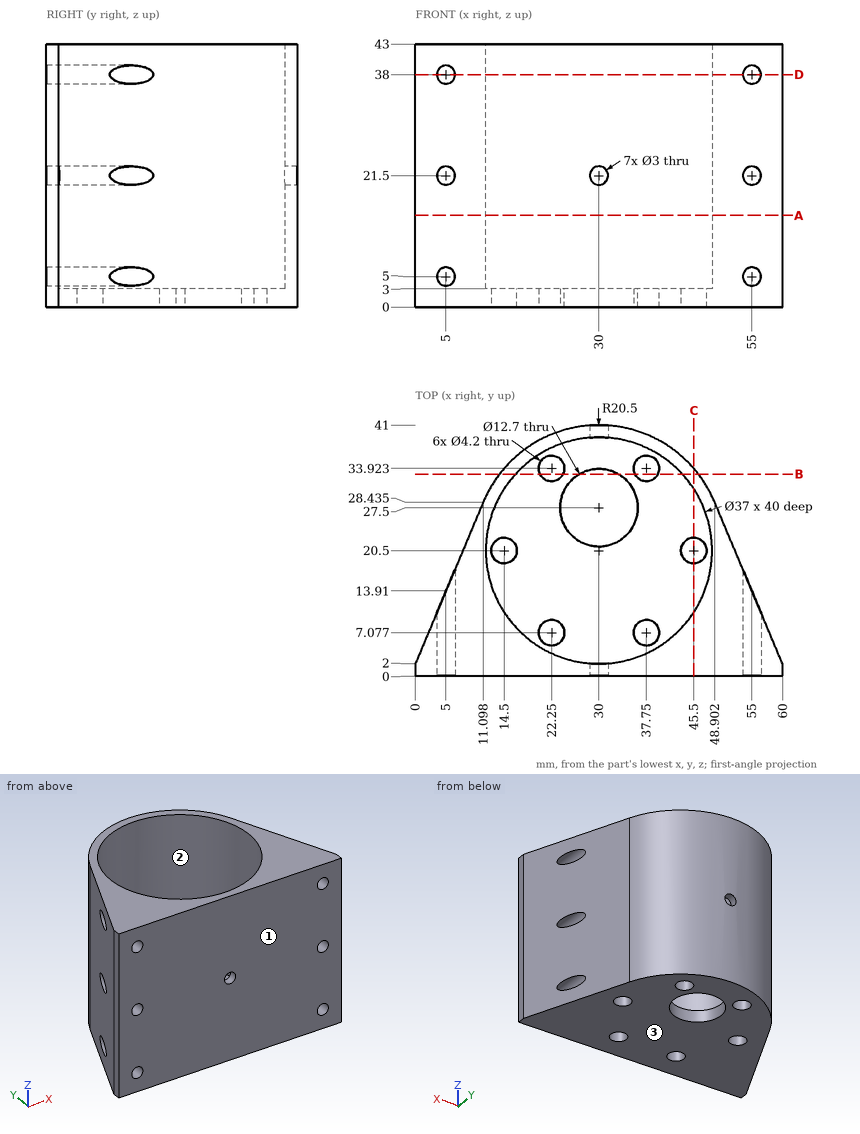
Design review of the part shown in the three views and the two pictorial views. Dimensions are in mm from the part's minimum x, y and z. Round coordinates to 2 decimals unless told otherwise and drop trailing zeros. Loops run counter-clockwise (first coordinate to the right, second up) from the corner with the lowest first, then second, coordinate; pieces in that order, holes last. Notation, with made-up numbers: M 48.5,-21 L 66.5,-21 A34 cw 66.5,16 Z; hole C 7,88 d6. An arc over 180 degrees is marked long. Put each result on its own line as item: value.
Q1. Consider section C-C, the plane x = 45.5. Give the boundary of the cut face in (y, z), then the cut area to 3 significant figures.
Result set:
outline: M 0,0 L 18.4,0 L 18.4,3 L 10.4,3 L 10.4,43 L 0,43 Z; M 22.6,0 L 33.92,0 L 33.92,43 L 30.6,43 L 30.6,3 L 22.6,3 Z
area: 638 mm²
Q2. Consider section B-B, the plane y = 33. Give the boundary of the cut face in (x, z).
Result set:
outline: M 13.75,0 L 20.36,0 L 20.36,3 L 16.36,3 L 16.36,43 L 13.75,43 Z; M 24.14,0 L 26.83,0 L 26.83,3 L 24.14,3 Z; M 33.17,0 L 35.86,0 L 35.86,3 L 33.17,3 Z; M 39.64,0 L 46.25,0 L 46.25,43 L 43.64,43 L 43.64,3 L 39.64,3 Z
Q3. To check wall thickness, follow L1, parallel to Z at x = 55, y = 11; L2, parallel to X at y = 5, z = 37 (1 decimal); L3, parallel to X at y = 7.25, z = 21.5 (1 decimal). State the ranges of each line that lie inside material, in increasing order.
Result set:
L1: z = 0 to 3.5, 6.5 to 20, 23 to 36.5, 39.5 to 43
L2: x = 1.3 to 3.9, 6.1 to 19.9, 40.1 to 53.9, 56.1 to 58.7
L3: x = 2.2 to 3.5, 6.5 to 17.1, 42.9 to 53.5, 56.5 to 57.8
Q4. Consider section A-A, the plane z = 15. Give the boundary of the cut face in (x, y) (1 decimal).
Result set:
outline: M 0,0 L 60,0 L 60,2 L 48.9,28.4 A20.5 ccw 11.1,28.4 L 0,2 Z; hole C 30,20.5 d37
Q5. Consider section D-D, the plane z = 38. Give the boundary of the cut face in (x, y) (1 decimal), then the cut area to 3 significant figures.
Result set:
outline: M 0,0 L 3.5,0 L 3.5,10.3 L 0,2 Z; M 6.5,0 L 53.5,0 L 53.5,17.5 L 48.9,28.4 A20.5 ccw 11.1,28.4 L 6.5,17.5 Z; M 56.5,0 L 60,0 L 60,2 L 56.5,10.3 Z; hole C 30,20.5 d37
area: 597 mm²
Q6. For pin 1 (11 mm diameter, centred on x = 35, y = 27, fed in from +Z); pin 2 (3 mm diameter, centred on y = 15, z = 20.5, fed in from +X); pin 3 (10 mm diameter, centred on x = 21, z = 32.5, fed in from +Y), all flat-tipped, find the tip position at first contact; note any pin that passes through.
Result set:
pin 1: stops at z = 3
pin 2: stops at x = 55.14
pin 3: stops at y = 40.61
Q7. Mouldability with a two-part tool opening along Y and no side actions: class the marked faces 1, 2 and 3 as released by +Y, released by -Y, zero draft, split by the parting line, or undercut.
Result set:
face 1: released by -Y
face 2: undercut
face 3: zero draft
